Build history of the part. All positions in model axes, mm. A direction names the side the tool comes from. Give positions to 0.01 mm unless a question says otherwise; leave off trailing zeros. Loops run counter-clockwise (first coordinate to the right, second up) from the corner with the lowest first, then second, coordinate; pieces in that order, holes last. Notation, with made-up numbers: M 43.5,-16.5 L 79.5,-16.5 A25 ccw 79.5,9.5 Z; hole C 11,10.25 d1. An arc over 180 degrees is marked long. Put each result on its own line as item: value.
```python
from build123d import *

# Parameters (mm, degrees)
SKETCH1_W           = 40.015172748
SKETCH1_H           = 40.015172748
BOSS_EXTRUDE1_DEPTH = 20
SKETCH1_3_R         = 8.95
SKETCH1_3_R_2       = 7.5
BOSS_EXTRUDE2_DEPTH = 3.5
SKETCH1_4_R         = 7.5
CUT_EXTRUDE1_DEPTH  = 35.649776695
SKETCH1_5_W         = 22.4
SKETCH1_5_H         = 4.3
CUT_EXTRUDE2_DEPTH  = 6.7
SKETCH7_W           = 36.015172748
SKETCH7_H           = 36.015172748
CUT_EXTRUDE3_DEPTH  = 4


with BuildPart() as part:
    # Sketch1 → Boss-Extrude1 (new body)
    with BuildSketch(Plane.XY):
        Rectangle(SKETCH1_W, SKETCH1_H)
    extrude(amount=BOSS_EXTRUDE1_DEPTH)

    # Sketch1<3> → Boss-Extrude2 (add)
    with BuildSketch(Plane.XY):
        Circle(SKETCH1_3_R)
        Circle(SKETCH1_3_R_2, mode=Mode.SUBTRACT)
    extrude(amount=-BOSS_EXTRUDE2_DEPTH)

    # Sketch1<4> → Cut-Extrude1 (cut, through all)
    with BuildSketch(Plane.XY):
        Circle(SKETCH1_4_R)
    extrude(amount=CUT_EXTRUDE1_DEPTH, mode=Mode.SUBTRACT)

    # Sketch1<5> → Cut-Extrude2 (cut)
    with BuildSketch(Plane.XY):
        with Locations((-0.1, -16.357586374)):
            Rectangle(SKETCH1_5_W, SKETCH1_5_H)
        with Locations((-0.1, 16.557586374)):
            Rectangle(SKETCH1_5_W, SKETCH1_5_H)
    extrude(amount=CUT_EXTRUDE2_DEPTH, mode=Mode.SUBTRACT)

    # Sketch7 → Cut-Extrude3 (cut)
    with BuildSketch(Plane.XY.offset(20)):
        Rectangle(SKETCH7_W, SKETCH7_H)
    extrude(amount=-CUT_EXTRUDE3_DEPTH, mode=Mode.SUBTRACT)


solid = part.part
```
Q1. Tool access for faces 1 (the flat face through (0, 8, 16)), 2 (the flat face through (11.1, -16, 3)), 3 (the cylindrical face through (-7.493, 0.33, 6.114)): list every direction of +Z, -Z, +X, -X, +Y, -Y with a clear straight run to the whole face (end or side of a thin tool).
Here are the results:
face 1: +Z
face 2: -Z
face 3: +Z, -Z
Q2. Slice it at D-D (z = 8.25). List the corners of the cut face in (x, y), and give its area (3 significant figures).
Here are the results:
outline: M -20.01,-20.01 L 20.01,-20.01 L 20.01,20.01 L -20.01,20.01 Z; hole C 0,0 d15
area: 1,420 mm²
Q3. Slice it at B-B (y = 0). List the corners of the cut face in (x, z).
Here are the results:
outline: M -20.01,0 L -8.95,0 L -8.95,-3.5 L -7.5,-3.5 L -7.5,16 L -18.01,16 L -18.01,20 L -20.01,20 Z; M 7.5,-3.5 L 8.95,-3.5 L 8.95,0 L 20.01,0 L 20.01,20 L 18.01,20 L 18.01,16 L 7.5,16 Z
Q4. Drop flat-ended pins along their axis: pin 1 Ø1.5 at (x, y) = (6.5, -9) entering from -Z; pin 2 Ø1.3 at (x, y) = (1.5, -16.5) entering from -Z; pin 3 Ø11 at (x, y) = (-2.5, 6) entering from +Z. Give the stop position or say it passes through.
Here are the results:
pin 1: z = 0
pin 2: z = 6.7
pin 3: z = 16
Q5. Slice it at A-A (z = 3.5). List the corners of the cut face in (x, y).
Here are the results:
outline: M -20.01,-20.01 L 20.01,-20.01 L 20.01,20.01 L -20.01,20.01 Z; hole M -11.3,-18.51 L 11.1,-18.51 L 11.1,-14.21 L -11.3,-14.21 Z; hole M -11.3,14.41 L 11.1,14.41 L 11.1,18.71 L -11.3,18.71 Z; hole C 0,0 d15
Q6. Probe line 1 (Y direction, x = 9, z = 4.75); line 2 (Y direction, x = 0, z = 3); line 3 (X direction, y = 0, z = 6). List the from-to ranges inside material, lowest first. Write a range as from..to.
Here are the results:
line 1: -20.01..-18.51, -14.21..14.41, 18.71..20.01
line 2: -20.01..-18.51, -14.21..-7.5, 7.5..14.41, 18.71..20.01
line 3: -20.01..-7.5, 7.5..20.01
Q7. Mould opens along X. For faces 4 (the flat face through (0, -16, 6.7)), 5 (the flat face through (-2, -19, 20)), 6 (the cylindrical face through (-7.1, -5.45, -1.73)) say: pulls with the +X half, pulls with the -X half, needs draft (parallel to the pull), parting line crosses it, or undercut.
Here are the results:
face 4: undercut
face 5: needs draft
face 6: parting line crosses it
Q8. Slice it at C-C (x = 0). List the corners of the cut face in (y, z), and give its area (3 significant figures).
Here are the results:
outline: M -20.01,0 L -18.51,0 L -18.51,6.7 L -14.21,6.7 L -14.21,0 L -8.95,0 L -8.95,-3.5 L -7.5,-3.5 L -7.5,16 L -18.01,16 L -18.01,20 L -20.01,20 Z; M 7.5,-3.5 L 8.95,-3.5 L 8.95,0 L 14.41,0 L 14.41,6.7 L 18.71,6.7 L 18.71,0 L 20.01,0 L 20.01,20 L 18.01,20 L 18.01,16 L 7.5,16 Z
area: 369 mm²
